Could you check a few things on this model? Use its own coordinates, in mm. Face numbers are marked on the shaded views. A direction names the side the tool comes from. Give positions to 0.01 mm unless a question says otherwise; leave off trailing zeros. Write each loop counter-clockwise with the first axis right and the second up, starting at its lowest first coordinate (ties: lowest second). Pieces come first, ordered by that corner, then holes. Notation, with made-up numbers: M -8.5,19.25 L 21.5,19.25 A20 cw 21.5,58.25 Z; hole C -28,40 d4. An arc over 180 degrees is marked long. Use one line per item in the form item = value.
from build123d import *

# Parameters (mm, degrees)
F0_R     = 25
F0_R_2   = 10
F1_DEPTH = 3
F2_DEPTH = 10
F3_D     = 5.5
F3_DEPTH = 30
F3_TIP   = 1.6523667023
F4_R     = 6.6209049639
F5_DEPTH = 5


with BuildPart() as f1:
    # F0 (on Top) → F1 (new body)
    with BuildSketch(Plane.XY):
        Circle(F0_R)
        Circle(F0_R_2, mode=Mode.SUBTRACT)
        Circle(F0_R_2)
    extrude(amount=F1_DEPTH)

    # F0 (on Top) → F2 (join)
    with BuildSketch(Plane.XY):
        Circle(F0_R_2)
    extrude(amount=F2_DEPTH)

    # F3
    with Locations(Plane(origin=(0, 0, 0), x_dir=(1, 0, 0), z_dir=(0, 0, -1))):
        with Locations((0, 0)):
            Hole(F3_D / 2, depth=F3_DEPTH)
            with Locations((0, 0, -(F3_DEPTH + F3_TIP / 2))):  # 118° drill point
                Cone(0, F3_D / 2, F3_TIP, mode=Mode.SUBTRACT)

    # F4 (on face) → F5 (cut)
    with BuildSketch(Plane.XY):
        Circle(F4_R)
        Polygon((-4.8497422612, 0), (-2.4248711306, 4.2), (2.4248711306, 4.2), (4.8497422612, 0), (2.4248711306, -4.2), (-2.4248711306, -4.2), align=None, mode=Mode.SUBTRACT)
        Polygon((2.4248711306, 4.2), (-2.4248711306, 4.2), (-4.8497422612, 0), (-2.4248711306, -4.2), (2.4248711306, -4.2), (4.8497422612, 0), align=None)
    extrude(amount=F5_DEPTH, mode=Mode.SUBTRACT)


solid = f1.part
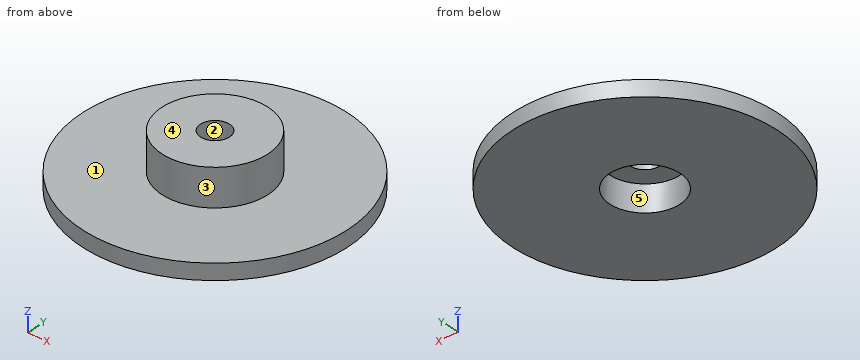
1) I want a section at C-C, the plane x = 6. Please give me the cut outline in (y, z), plus the area to 3 significant figures.
Checked values:
outline = M -24.27,0 L -2.8,0 L -2.8,5 L 2.8,5 L 2.8,0 L 24.27,0 L 24.27,3 L 8,3 L 8,10 L -8,10 L -8,3 L -24.27,3 Z
area = 230 mm2
2) Thinking about a two-plate mould opening in Y: for the marked faces 1, 2 and 3, which applies, released by +Y, released by -Y, zero draft, split by the parting line, or undercut?
Checked values:
face_1 = zero draft
face_2 = undercut
face_3 = split by the parting line
3) I want a section at A-A, the plane x = 0. Please give me the cut outline in (y, z), plus the area to 3 significant figures.
Checked values:
outline = M -25,0 L -6.62,0 L -6.62,5 L -2.75,5 L -2.75,10 L -10,10 L -10,3 L -25,3 Z; M 2.75,5 L 6.62,5 L 6.62,0 L 25,0 L 25,3 L 10,3 L 10,10 L 2.75,10 Z
area = 196 mm2
4) For pin 1 Ø4 at (x, y) = (7.5, 19) entering from +Z; pin 2 Ø4.5 at (x, y) = (0, 0) entering from -Z; pin 3 Ø4 at (y, z) = (-6.5, 2) entering from -X; pin 4 Ø5 at (x, z) = (-17.5, 2) entering from +Y, each with a flat end and sliding along its axis, tell me the tip position at first contact or that it passes through.
Checked values:
pin_1 = 3
pin_2 = through
pin_3 = -24.59
pin_4 = 20
5) For the marked faces 4 and 5, which set-ups out of +Z, -Z, +X, -X, +Y, -Y let a thin tool reach every point of the face, with its end or its side?
Checked values:
face_4 = +Z, +X, -X, +Y, -Y
face_5 = -Z
6) I want a section at D-D, the plane y = -8. Please give me the cut outline in (x, z), plus the area to 3 significant figures.
Checked values:
outline = M -23.69,0 L 23.69,0 L 23.69,3 L 6,3 L 6,10 L -6,10 L -6,3 L -23.69,3 Z
area = 226 mm2
7) If I drill on L1, parallel to Y at x = 0, z = 6.4; L2, parallel to Y at x = 0, z = 1; L3, parallel to X at y = -6, z = 2.5, over which ranges is the centre line in solid material (lowest first)?
Checked values:
L1 = -10 to -2.75, 2.75 to 10
L2 = -25 to -6.62, 6.62 to 25
L3 = -24.27 to -2.8, 2.8 to 24.27
